```python
from build123d import *

# Parameters (mm, degrees)
F0_W     = 82.4639983475
F0_H     = 48.5082380474
F1_DEPTH = 25.4
F2_W     = 13.8226579875
F2_H     = 35.7262613252
F3_DEPTH = 5.08
F4_R     = 5.07999


# Not quite as in the source:
# - a fillet or chamfer is up to 0.001 mm smaller than in the source, because OpenCascade refuses the exact size


with BuildPart() as f1:
    # F0 (on Front) → F1 (new body)
    with BuildSketch(Plane.XZ):
        with Locations((4.3657366186, -4.1232034564)):
            Rectangle(F0_W, F0_H)
    extrude(amount=F1_DEPTH)

    # F2 (on face) → F3 (join)
    with BuildSketch(Plane(origin=(-36.8662625551, 0, 0), x_dir=(0, -1, 0), z_dir=(-1, 0, 0))):
        with Locations((12.4125434086, -4.4842208736)):
            Rectangle(F2_W, F2_H)
    extrude(amount=F3_DEPTH)

    # F4 (radius 5.08 in the source; OpenCascade refuses exactly that, so slightly less here)
    f4_edges = [f1.edges().sort_by_distance(p)[0] for p in [
        (-41.946263, -12.412543, -22.347352),
        (-41.946263, -5.501214, -4.484221),
        (-41.946263, -19.323872, -4.484221),
        (-41.946263, -12.412543, 13.37891),
    ]]
    fillet(f4_edges, radius=F4_R)


solid = f1.part
```
Read the model definition and answer for the solid it produces. Units are mm, in the model's axes. Coordinates: 2 decimals unless noted, no trailing zeros. Order: outer loops, then holes, each group sorted by start corner. A loop starts at its lowest first (then second) coordinate and runs counter-clockwise, first axis right, second up. Notation, with made-up numbers: (70, 64.5) - (122, 64.5) arc R35 cw to (122, 102.5) - close; hole circle Ø10 at (22.25, 65.25). An arc over 180 degrees is marked (long way). Answer as a JSON object with one key per item and string values. Group by question number.
Item 1: Section B-B (y = -20.5) is taken. Give the vertices of the cut face in (x, z).
Item 2: Section D-D (z = 17) is taken. Give the vertices of the cut face in (x, y).
Item 3: Consider probe 1 along X at (y, z) = (-2.5, -8.5); probe 2 along X at (y, z) = (-10.25, -4); probe 3 along Z at (x, y) = (-37, -17.5). Determine where each line is inside the solid, lowest interval first. Write a range as from..to.
Results are:
{
 "1": {"outline": "(-36.87, -28.38) - (45.6, -28.38) - (45.6, 20.13) - (-36.87, 20.13) - close"},
 "2": {"outline": "(-36.87, -25.4) - (45.6, -25.4) - (45.6, 0) - (-36.87, 0) - close"},
 "3": {"probe 1": "x = -36.87..45.6", "probe 2": "x = -41.94..45.6", "probe 3": "z = -22.35..13.38"}
}
